```python
from build123d import *

# Parameters (mm, degrees)
F0_W   = 1.85994
F0_H   = 1
F0_H_2 = 1.5
F2_R   = 0.8


with BuildPart() as f1:
    # F0 (on Front) → F1 (revolve)
    with BuildSketch(Plane.XZ):
        Polygon((-28.14006, 0), (0, 0), (28.14006, 0), (28.14006, 1), (-28.14006, 1), align=None)
        with Locations((29.07003, -0.5)):
            Rectangle(F0_W, F0_H)
        with Locations((-29.07003, 0.5)):
            Rectangle(F0_W, F0_H)
        with Locations((29.07003, 1.75)):
            Rectangle(F0_W, F0_H_2)
        with Locations((-29.07003, 1.75)):
            Rectangle(F0_W, F0_H_2)
    revolve(axis=Axis((0, 0, 0), (-1, 0, 0)))

    # F2
    f2_edges = [f1.edges().sort_by_distance(p)[0] for p in [
        (-30, 0, -2.5),
        (30, 0, -2.5),
    ]]
    fillet(f2_edges, radius=F2_R)


solid = f1.part
```
Can you work these out from the model? Positions are in its coordinate system, mm. A direction names the side the tool comes from. Round coordinates to 2 decimals unless told otherwise and drop trailing zeros. Loops run counter-clockwise (first coordinate to the right, second up) from the corner with the lowest first, then second, coordinate; pieces in that order, holes last. Notation, with made-up numbers: (26.25, 47) -> (75.25, 47) arc R26 cw to (75.25, 61) -> close; hole circle Ø8 at (-28, 16.5). An arc over 180 degrees is marked (long way). Answer in a Markdown table with one row per item.
Item 1: Suppose I cut it at A-A, the plane z = 0. List the corners of the cut face in (x, y) for me, plus the area to 3 significant figures.
Answer block:
| item | result |
|---|---|
| outline | (-30, -1.7) arc R0.8 ccw to (-29.2, -2.5) -> (-28.14, -2.5) -> (-28.14, -1) -> (28.14, -1) -> (28.14, -2.5) -> (29.2, -2.5) arc R0.8 ccw to (30, -1.7) -> (30, 1.7) arc R0.8 ccw to (29.2, 2.5) -> (28.14, 2.5) -> (28.14, 1) -> (-28.14, 1) -> (-28.14, 2.5) -> (-29.2, 2.5) arc R0.8 ccw to (-30, 1.7) -> close |
| area | 131 mm² |
Item 2: Will these pins go through, and if not, where does the flat tip stop? P1, Ø1, axis at x = -15, z = -1, coming from the -Y side; P2, Ø3, axis at x = 7.5, z = -1.5, coming from the +Y side; P3, Ø3, axis at x = -3, y = 1.5, coming from the -Z side.
Answer block:
| item | result |
|---|---|
| P1 | y = -0.87 |
| P2 | y = 1 |
| P3 | z = -1 |
Item 3: On a 3-axis mill with a long thin cutter (end or side, diameter ignored), from which of +Z, -Z, +X, -X, +Y, -Y can I reach the whole of each face in a straight line? I mean faces 1 (the cylindrical face through (28.68, -2.44, -0.54)), 2 (the cylindrical face through (0, -1, 0)). Say none if no direction works.
Answer block:
| item | result |
|---|---|
| face 1 | +X, -X |
| face 2 | none |
Item 4: If I drill on probe 1 along X at (y, z) = (0.5, 1.35); probe 2 along X at (y, z) = (0, 2.2); probe 3 along Y at (x, z) = (15, -0.05), over which ranges is the centre line in solid material (lowest first)?
Answer block:
| item | result |
|---|---|
| probe 1 | -30 to -28.14, 28.14 to 30 |
| probe 2 | -29.82 to -28.14, 28.14 to 29.82 |
| probe 3 | -1 to 1 |
Item 5: We'd pull the mould along X, two halves only. Please class faces 3 (the flat face through (-30, 0, 0)), 4 (the flat face through (30, 0, 0)), 5 (the cylindrical face through (-28.66, -2.44, -0.54)), 6 (the flat face through (-28.14, -1, -1)): released by +X, released by -X, zero draft, split by the parting line, or undercut.
Answer block:
| item | result |
|---|---|
| face 3 | released by -X |
| face 4 | released by +X |
| face 5 | zero draft |
| face 6 | undercut |
Item 6: Suppose I cut it at C-C, the plane x = -22.5. List the corners of the cut face in (y, z) for me, plus the area to 3 significant figures.
Answer block:
| item | result |
|---|---|
| outline | circle Ø2 at (0, 0) |
| area | 3.14 mm² |
